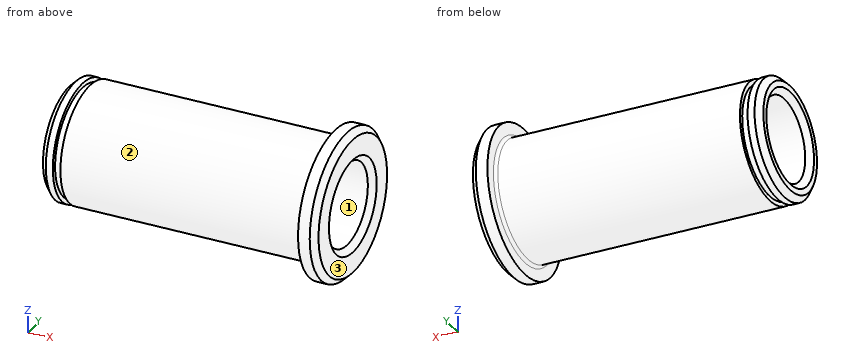
from build123d import *

# Parameters (mm, degrees)
CHAMFER1_SIZE = 1
FILLET1_R     = 0.5


with BuildPart() as part:
    # Sketch1 → Revolve1 (revolve)
    with BuildSketch(Plane.XY, mode=Mode.PRIVATE) as revolve1_sk:
        Polygon((0, -7), (48.5, -7), (48.5, -12.5), (45.5, -12.5), (45.5, -10), (3.5, -10), (3.5, -9.25), (2.2, -9.25), (2.2, -10), (0, -10), align=None)
    revolve(revolve1_sk.sketch.rotate(Axis((0, 0, 0), (1, 0, 0)), 270), axis=Axis((0, 0, 0), (1, 0, 0)))

    # Chamfer1
    chamfer1_edges = [part.edges().sort_by_distance(p)[0] for p in [
        (48.5, 0, -12.5),
        (48.5, 0, -7),
        (0, 0, -7),
        (0, 0, -10),
    ]]
    chamfer(chamfer1_edges, length=CHAMFER1_SIZE)

    # Fillet1
    fillet1_edges = [part.edges().sort_by_distance(p)[0] for p in [
        (45.5, 0, -10),
    ]]
    fillet(fillet1_edges, radius=FILLET1_R)


solid = part.part
Design review of the part built by this model. Coordinates are the model's own, in mm. Face numbers are marked on the shaded views. Coordinates: 2 decimals unless noted, no trailing zeros. Order: outer loops, then holes, each group sorted by start corner. A loop starts at its lowest first (then second) coordinate and runs counter-clockwise, first axis right, second up.
Item 1: For line 1 (Y direction, x = 31.5, z = -4.75); line 2 (Y direction, x = 29, z = -6.25); line 3 (X direction, y = -0.25, z = 11), list the stretches that pass through material, from the lowest coordinate up.
Item 2: Take a section at C-C, the plane x = 19.5. Write out the cut boundary in (y, z), then the cut area to 3 significant figures.
Item 3: For pin 1 Ø8 at (x, z) = (12, 0.5) entering from +Y; pin 2 Ø10 at (x, z) = (25.5, -8) entering from +Y; pin 3 Ø6 at (x, z) = (36, -4) entering from +Y, all flat-tipped, find the tip position at first contact; note any pin that passes through.
Item 4: The part is to be moulded in two halves that separate along Z. For the marked faces 1, 2 and 3, say which applies: pulls with the +Z half, pulls with the -Z half, needs draft (parallel to the pull), parting line crosses it, or undercut.
The answers:
1. line 1: y = -8.8 to -5.14, 5.14 to 8.8
1. line 2: y = -7.81 to -3.15, 3.15 to 7.81
1. line 3: x = 45.5 to 48.5
2. outline: circle Ø20 at (0, 0); hole circle Ø14 at (0, 0)
2. area: 160 mm2
3. pin 1: stops at y = 10
3. pin 2: stops at y = 9.54
3. pin 3: stops at y = 9.95
4. face 1: undercut
4. face 2: parting line crosses it
4. face 3: needs draft
